For this review, take the finished solid that the model builds, in its own axes (mm). A direction names the side the tool comes from. Give positions to 0.01 mm unless a question says otherwise; leave off trailing zeros. Order: outer loops, then holes, each group sorted by start corner. A loop starts at its lowest first (then second) coordinate and runs counter-clockwise, first axis right, second up.
from build123d import *

# Parameters (mm, degrees)
SKETCH_1_W      = 4
SKETCH_1_H      = 16.4
EXTRUDE_1_DEPTH = 9
SKETCH_2_R      = 4.5
SKETCH_2_R_2    = 1.6
EXTRUDE_2_DEPTH = 4
FILLET_1_R      = 4
FILLET_2_R      = 1.6
CHAMFER_1_SIZE  = 0.2


with BuildPart() as part:
    # 草图1 → 凸台-拉伸1 (new body)
    with BuildSketch(Plane(origin=(0, 0, 0), x_dir=(1, 0, 0), z_dir=(0, 1, 0))):
        Polygon((106.5, 0), (0, 0), (0, -4), (110.5, -4), (110.5, 38), (0, 38), (0, 34), (106.5, 34), align=None)
        with Locations((112.5, 29.8)):
            Rectangle(SKETCH_1_W, SKETCH_1_H)
        with Locations((112.5, 4.2)):
            Rectangle(SKETCH_1_W, SKETCH_1_H)
    extrude(amount=EXTRUDE_1_DEPTH)

    # 草图2 → 凸台-拉伸2 (add)
    # profile 1 of 6: a face of its own
    with BuildSketch(Plane.ZY):
        with Locations((-42.5, 4.5)):
            Circle(SKETCH_2_R)
        with Locations((-42.5, 4.5)):
            Circle(SKETCH_2_R_2, mode=Mode.SUBTRACT)
    # profile 2 of 6: a face of its own
    with BuildSketch(Plane.ZY):
        with BuildLine():
            Line((-38, 9), (-42.5, 9))
            ThreePointArc((-42.5, 9), (-39.318019485, 7.681980515), (-38, 4.5))
            Line((-38, 4.5), (-38, 9))
        make_face()
    # profile 3 of 6: a face of its own
    with BuildSketch(Plane.ZY):
        with BuildLine():
            ThreePointArc((-38, 4.5), (-39.318019485, 1.318019485), (-42.5, 0))
            Line((-42.5, 0), (-38, 0))
            Line((-38, 0), (-38, 4.5))
        make_face()
    # profile 4 of 6: a face of its own
    with BuildSketch(Plane.ZY):
        with Locations((8.5, 4.5)):
            Circle(SKETCH_2_R)
        with Locations((8.5, 4.5)):
            Circle(SKETCH_2_R_2, mode=Mode.SUBTRACT)
    # profile 5 of 6: a face of its own
    with BuildSketch(Plane.ZY):
        with BuildLine():
            Line((8.5, 9), (4, 9))
            Line((4, 9), (4, 4.499999989))
            ThreePointArc((4, 4.499999989), (5.318019481, 7.681980511), (8.5, 9))
        make_face()
    # profile 6 of 6: a face of its own
    with BuildSketch(Plane.ZY):
        with BuildLine():
            ThreePointArc((8.5, 0), (5.318019489, 1.318019481), (4, 4.499999989))
            Line((4, 4.499999989), (4, 0))
            Line((4, 0), (8.5, 0))
        make_face()
    extrude(amount=-EXTRUDE_2_DEPTH)

    # 圆角1
    fillet_1_edges = [part.edges().sort_by_distance(p)[0] for p in [
        (0, 4.5, -34),
        (114.5, 4.5, -38),
        (114.5, 4.5, 4),
        (0, 4.5, 0),
    ]]
    fillet(fillet_1_edges, radius=FILLET_1_R)

    # 圆角2
    fillet_2_edges = [part.edges().sort_by_distance(p)[0] for p in [
        (106.5, 4.5, 0),
        (106.5, 4.5, -34),
        (114.5, 4.5, -21.6),
        (114.5, 4.5, -12.4),
        (4, 4.5, -38),
        (4, 4.5, 4),
    ]]
    fillet(fillet_2_edges, radius=FILLET_2_R)

    # 倒角1
    chamfer_1_edges = [part.edges().sort_by_distance(p)[0] for p in [
        (111.7, 0, -12.4),
        (111.7, 9, -12.4),
        (58.05, 0, -38),
        (111.7, 0, -21.6),
        (54.45, 0, 0),
        (106.5, 0, -17),
        (114.03137085, 0, -22.06862915),
        (114.03137085, 0, -11.93137085),
        (58.05, 9, -38),
        (4, 9, -41.05),
        (106.5, 9, -17),
        (54.45, 9, 0),
        (4, 9, 7.05),
        (111.7, 9, -21.6),
        (114.03137085, 9, -22.06862915),
        (114.03137085, 9, -11.93137085),
        (4.46862915, 9, 4.46862915),
        (4.46862915, 0, 4.46862915),
        (4.46862915, 0, -38.46862915),
        (4.46862915, 9, -38.46862915),
        (106.03137085, 0, -0.46862915),
        (106.03137085, 9, -0.46862915),
        (106.03137085, 0, -33.53137085),
        (106.03137085, 9, -33.53137085),
        (110.5, 0, -17),
        (110.5, 9, -17),
        (0, 4.5, -47),
        (4, 0, -41.05),
        (4, 4.5, -47),
        (4, 4.5, 13),
        (4, 0, 7.05),
        (0, 4.5, 13),
        (54.45, 0, -34),
        (0, 0, -40.25),
        (114.5, 0, -28.6),
        (114.5, 0, -5.4),
        (58.05, 0, 4),
        (0, 0, 6.25),
        (1.171572875, 0, -35.171572875),
        (1.171572875, 0, 1.171572875),
        (113.328427125, 0, 2.828427125),
        (113.328427125, 0, -36.828427125),
        (114.5, 9, -28.6),
        (0, 9, 6.25),
        (58.05, 9, 4),
        (114.5, 9, -5.4),
        (0, 9, -40.25),
        (54.45, 9, -34),
        (1.171572875, 9, -35.171572875),
        (1.171572875, 9, 1.171572875),
        (113.328427125, 9, 2.828427125),
        (113.328427125, 9, -36.828427125),
    ]]
    chamfer(chamfer_1_edges, length=CHAMFER_1_SIZE)


solid = part.part
1) Tool access review of faces 4 (the face through (1.141, 4.56, 1.203)), 5 (the face through (110.5, 4, -17)), 6 (the face through (4, 3.6, -44.1)): name each direction out of +Z, -Z, +X, -X, +Y, -Y from which nothing blocks a thin tool from reaching the whole face with its end or side.
Answer sheet:
face 4: -X, +Y, -Y
face 5: +X, +Y, -Y
face 6: -Z, +X, +Y, -Y
2) We need section C-C on z = -5. Give the boundary of the cut face in (x, y), then the cut area to 3 significant figures.
Answer sheet:
outline: (106.5, 0.2) - (106.7, 0) - (114.3, 0) - (114.5, 0.2) - (114.5, 8.8) - (114.3, 9) - (106.7, 9) - (106.5, 8.8) - close
area: 71.9 mm2
3) To check wall thickness, follow line 1 (Z direction, x = 28, y = 8.25); line 2 (Z direction, x = 107.5, y = 0.75); line 3 (Y direction, x = 2, z = -42.5). State the ranges of each line that lie inside material, in increasing order.
Answer sheet:
line 1: z = -38 to -34, 0 to 4
line 2: z = -38 to 4
line 3: y = 0 to 2.9, 6.1 to 9
4) We need section B-B on y = 4.5. Count the separate pieces of the cut face and the enclosed holes in it, then the cut area to 3 significant figures.
Answer sheet:
separate pieces: 3
enclosed holes: 0
area: 1,180 mm2
5) Clearance check with flat-ended pins moving along their axes: pin 1 (2.5 mm diameter, centred on y = 6.5, z = -17.5, fed in from -X); pin 2 (1.2 mm diameter, centred on x = 111.5, y = 6.5, fed in from -Z); pin 3 (5 mm diameter, centred on y = 3, z = -18, fed in from +X). State where each tip first meets the part, or that it passes through.
Answer sheet:
pin 1: stops at x = 106.5
pin 2: stops at z = -37.98
pin 3: stops at x = 110.5
6) Draft analysis for pull direction Y (two halves, no side actions). For faces 1 (the face through (70, 9, -36)), 2 (the face through (54, 4, -34)), 3 (the face through (1.97, 2.94, -42.85)), state which applies: +Y half, -Y half, draft (parallel to the pull), parting line (faces both ways), or undercut.
Answer sheet:
face 1: +Y half
face 2: draft
face 3: undercut
7) We need section A-A on x = 66. Give the boundary of the cut face in (y, z), then the cut area to 3 significant figures.
Answer sheet:
outline: (0, -37.8) - (0.2, -38) - (8.8, -38) - (9, -37.8) - (9, -34.2) - (8.8, -34) - (0.2, -34) - (0, -34.2) - close; (0, 0.2) - (0.2, 0) - (8.8, 0) - (9, 0.2) - (9, 3.8) - (8.8, 4) - (0.2, 4) - (0, 3.8) - close
area: 71.8 mm2
